Source: CAD feature listing. Evaluate the final solid. Frame: model axes, mm. A direction names the side the tool comes from. Give positions to 0.01 mm unless a question says otherwise; leave off trailing zeros. Loops run counter-clockwise (first coordinate to the right, second up) from the corner with the lowest first, then second, coordinate; pieces in that order, holes last.
from build123d import *

# Parameters (mm, degrees)
SKETCH1_R                     = 11
BOSS_BASE_FLANGE_DEPTH        = 2
BOSS_BASE_FLANGE_TAPER        = 45
SKETCH2_R                     = 9
BOSS_SPECTRA_SPOOL_DEPTH      = 13
SKETCH3_R                     = 9
BOSS_TOP_FLANGE_DEPTH         = 2
BOSS_TOP_FLANGE_DRAFT         = -45
SKETCH4_R                     = 11
BOSS_TOP_EXTENSION_DEPTH      = 8
SKETCH5_R                     = 2.6
CUT_STEPPER_SHAFT_DEPTH       = 30.444863729
CUT_SET_SCREW_HOLE_REACH      = 37.071
CUT_SET_SCREW_HOLE_END_RADIUS = 2.6
SKETCH7_R                     = 1.75
SKETCH8_R                     = 3.1
CUT_SCREW_HEAD_SLOT_DEPTH     = 2
CUT_FLATEN_REACH              = 31.445
SKETCH6_W                     = 0.753049234
SKETCH6_H                     = 8
CUT_NUT_HOLE_DEPTH            = 5
SKETCH11_W                    = 3.354551733
SKETCH11_H                    = 5.7
CUT_NUT_SLOT_DEPTH            = 5
CIRPATTERN1_COUNT             = 3
CUT_THREAD_HOLE_DEPTH         = 30.444863729
SKETCH15_W                    = 1.5
SKETCH15_H                    = 1
CUT_EXTRUDE8_DEPTH            = 28.81186797
CHAMFER1_SIZE                 = 1
CHAMFER1_SIZE2                = 0.707106781
CHAMFER3_SIZE                 = 0.3
CHAMFER3_SIZE2                = 0.519615242
SKETCH16_OUTSIDE_W            = 31.982
SKETCH16_OUTSIDE_H            = 31.982
SKETCH16_OUTSIDE_R            = 10.5
CUT_TRUNCATE_BASE_DEPTH       = 5
SKETCH8_2_R                   = 3.1
CUT_EXTRUDE9_DEPTH            = 3


with BuildPart() as part:
    # Sketch1 → Boss-Base Flange (new body)
    with BuildSketch(Plane.XY):
        Circle(SKETCH1_R)
    extrude(amount=BOSS_BASE_FLANGE_DEPTH, taper=BOSS_BASE_FLANGE_TAPER)

    # Sketch2 → Boss-Spectra Spool (add)
    with BuildSketch(Plane.XY.offset(2)):
        with Locations(Location((0, 0, 0), (0, 0, 180))):
            Circle(SKETCH2_R)
    extrude(amount=BOSS_SPECTRA_SPOOL_DEPTH)


with BuildPart() as boss_top_flange_tool:
    # Sketch3 → Boss-Top Flange (with draft: the straight prism first)
    with BuildSketch(Plane.XY.offset(15)):
        with Locations(Location((0, 0, 0), (0, 0, 180))):
            Circle(SKETCH3_R)
    extrude(amount=BOSS_TOP_FLANGE_DEPTH)
    # Boss-Top Flange: the draft: its side faces are tilted about the plane it starts from
    boss_top_flange_sides = [boss_top_flange_tool.faces().sort_by_distance(p)[0] for p in [
        (9, 0, 16),
    ]]
    draft(boss_top_flange_sides, Plane.XY.offset(15), BOSS_TOP_FLANGE_DRAFT)


with BuildPart() as part_1:
    add(part.part)

    # Boss-Top Flange: add boss_top_flange_tool
    add(boss_top_flange_tool.part)

    # Sketch4 → Boss-Top Extension (add)
    with BuildSketch(Plane.XY.offset(17)):
        Circle(SKETCH4_R)
    extrude(amount=BOSS_TOP_EXTENSION_DEPTH)

    # Sketch5 → Cut-Stepper Shaft (cut, through all)
    with BuildSketch(Plane(origin=(0, 0, 0), x_dir=(-1, 0, 0), z_dir=(0, 0, -1))):
        Circle(SKETCH5_R)
    extrude(amount=-CUT_STEPPER_SHAFT_DEPTH, mode=Mode.SUBTRACT)

    # Cut-Set Screw Hole: up to this cylinder (the profile starts outside it)
    cut_set_screw_hole_end = Plane(origin=(0, 0, 20), z_dir=(0, 0, -1)) * Cylinder(CUT_SET_SCREW_HOLE_END_RADIUS, 80.342, mode=Mode.PRIVATE)
    # Sketch7 → Cut-Set Screw Hole (cut, up to the surface)
    with BuildSketch(Plane(origin=(-11, 0, 0), x_dir=(0, 0, -1), z_dir=(1, 0, 0)), mode=Mode.PRIVATE) as cut_set_screw_hole_sk1:
        with Locations(Location((-20, 0, 0), (0, 0, 180))):
            Circle(SKETCH7_R)
    cut_set_screw_hole_tool1 = extrude(cut_set_screw_hole_sk1.sketch, amount=CUT_SET_SCREW_HOLE_REACH, mode=Mode.PRIVATE) - cut_set_screw_hole_end
    cut_set_screw_hole = cut_set_screw_hole_tool1.solids().sort_by_distance((-11, 0, 20))[0]
    add(cut_set_screw_hole, mode=Mode.SUBTRACT)

    # Sketch8 → Cut-Screw Head Slot (cut)
    with BuildSketch(Plane(origin=(-11, 0, 0), x_dir=(0, 0, -1), z_dir=(1, 0, 0))):
        with Locations(Location((-20, 0, 0), (0, 0, 194.592594316))):
            Circle(SKETCH8_R)
    cut_screw_head_slot = extrude(amount=CUT_SCREW_HEAD_SLOT_DEPTH, mode=Mode.SUBTRACT)

    # Cut-Flaten: up to this cone (the profile starts inside it)
    cut_flaten_end = Plane(origin=(0, 0, 25), z_dir=(0, 0, 1)).offset(-18.999999) * Cone(1e-06, 69.945, 69.944999, align=(Align.CENTER, Align.CENTER, Align.MIN), mode=Mode.PRIVATE)
    # Sketch6 → Cut-Flaten (cut, up to the surface)
    with BuildSketch(Plane.XY.offset(25), mode=Mode.PRIVATE) as cut_flaten_sk1:
        with Locations((-10.623475383, 0)):
            Rectangle(SKETCH6_W, SKETCH6_H)
    cut_flaten_tool1 = extrude(cut_flaten_sk1.sketch, amount=-CUT_FLATEN_REACH, mode=Mode.PRIVATE) & cut_flaten_end
    cut_flaten = cut_flaten_tool1.solids().sort_by_distance((-10.623475, 0, 25))[0]
    add(cut_flaten, mode=Mode.SUBTRACT)

    # Sketch10 → Cut-Nut Hole (cut)
    with BuildSketch(Plane.ZY):
        Polygon((23.290896534, 0), (21.645448267, 2.85), (18.354551733, 2.85), (16.709103466, 0), (18.354551733, -2.85), (21.645448267, -2.85), align=None)
    cut_nut_hole = extrude(amount=CUT_NUT_HOLE_DEPTH, mode=Mode.SUBTRACT)

    # Sketch11 → Cut-Nut Slot (cut)
    with BuildSketch(Plane.ZY):
        with Locations((23.322724134, 0)):
            Rectangle(SKETCH11_W, SKETCH11_H)
    cut_nut_slot = extrude(amount=CUT_NUT_SLOT_DEPTH, mode=Mode.SUBTRACT)

    # CirPattern1: Cut-Set Screw Hole, Cut-Screw Head Slot, Cut-Flaten, Cut-Nut Hole, Cut-Nut Slot ×3 about axis
    cirpattern1_axis = Axis((0, 0, 0), (0, 0, 1))
    add([cut_set_screw_hole.rotate(cirpattern1_axis, i * 360 / CIRPATTERN1_COUNT) for i in range(1, CIRPATTERN1_COUNT)], mode=Mode.SUBTRACT)
    add([cut_screw_head_slot.rotate(cirpattern1_axis, i * 360 / CIRPATTERN1_COUNT) for i in range(1, CIRPATTERN1_COUNT)], mode=Mode.SUBTRACT)
    add([cut_flaten.rotate(cirpattern1_axis, i * 360 / CIRPATTERN1_COUNT) for i in range(1, CIRPATTERN1_COUNT)], mode=Mode.SUBTRACT)
    add([cut_nut_hole.rotate(cirpattern1_axis, i * 360 / CIRPATTERN1_COUNT) for i in range(1, CIRPATTERN1_COUNT)], mode=Mode.SUBTRACT)
    add([cut_nut_slot.rotate(cirpattern1_axis, i * 360 / CIRPATTERN1_COUNT) for i in range(1, CIRPATTERN1_COUNT)], mode=Mode.SUBTRACT)

    # Sketch13 → Cut-Thread Hole (cut, through all)
    with BuildSketch(Plane.XY.offset(25)):
        Polygon((-4.066025404, 1), (-4.932050808, 0.5), (-4.932050808, -0.5), (-4.066025404, -1), (-3.2, -0.5), (-3.2, 0.5), align=None)
    extrude(amount=-CUT_THREAD_HOLE_DEPTH, mode=Mode.SUBTRACT)

    # Sketch15 → Cut-Extrude8 (cut, symmetric)
    with BuildSketch(Plane(origin=(-5.5, 0, 5.5), x_dir=(0.7071067811865464, 0, 0.7071067811865488), z_dir=(-0.7071067811865488, 0, 0.7071067811865464))):
        with Locations((-4.189918951, 0)):
            Rectangle(SKETCH15_W, SKETCH15_H)
    cut_extrude8 = extrude(amount=CUT_EXTRUDE8_DEPTH, both=True, mode=Mode.SUBTRACT)

    # Chamfer1
    chamfer1_edges = [part_1.edges().sort_by_distance(p)[0] for p in [
        (-4.932050808, 0, 0.067270773),
    ]]
    chamfer1_side = [part_1.faces().sort_by_distance(p)[0] for p in [
        (-6.963711629, 0, 2.098931595),
    ]]
    chamfer(chamfer1_edges, length=CHAMFER1_SIZE, length2=CHAMFER1_SIZE2, reference=chamfer1_side[0])

    # Mirror1: Cut-Extrude8 across plane
    add(cut_extrude8.mirror(Plane.XY.offset(8.5)), mode=Mode.SUBTRACT)

    # Chamfer3
    chamfer3_edges = [part_1.edges().sort_by_distance(p)[0] for p in [
        (2.6, 0, 0),
    ]]
    chamfer3_side = [part_1.faces().sort_by_distance(p)[0] for p in [
        (-10.688873016, 0, 0),
    ]]
    chamfer(chamfer3_edges, length=CHAMFER3_SIZE, length2=CHAMFER3_SIZE2, reference=chamfer3_side[0])

    # Sketch16 outside → Cut-Truncate Base (cut)
    with BuildSketch(Plane(origin=(0, 0, 0), x_dir=(-1, 0, 0), z_dir=(0, 0, -1))):
        Rectangle(SKETCH16_OUTSIDE_W, SKETCH16_OUTSIDE_H)
        Circle(SKETCH16_OUTSIDE_R, mode=Mode.SUBTRACT)
    extrude(amount=-CUT_TRUNCATE_BASE_DEPTH, mode=Mode.SUBTRACT)

    # Sketch8<2> → Cut-Extrude9 (cut)
    with BuildSketch(Plane(origin=(-11, 0, 0), x_dir=(0, 0, -1), z_dir=(1, 0, 0))):
        with Locations((-20, 0)):
            Circle(SKETCH8_2_R)
    extrude(amount=CUT_EXTRUDE9_DEPTH, mode=Mode.SUBTRACT)


solid = part_1.part
1) Reachability of faces 1 (the flat face through (-3.2, 0, 9)), 2 (the flat face through (2.535, 4.31, 22.639)), 3 (the flat face through (-7, -0.5, 16)), 4 (the cylindrical face through (-9.139, -3.066, 19.543)) from +Z, -Z, +X, -X, +Y, -Y: full face, straight path, thin tool, end or side. Return the list, or none.
Checks:
face 1: +Z, -Z
face 2: +Z
face 3: none
face 4: -X
2) Contact query for flat-ended pins moving along their axis: P1, Ø7, axis at y = 0, z = 20, coming from the -X side; P2, Ø2, axis at x = -2.5, z = 19.5, coming from the +Y side; P3, Ø2, axis at y = 4.5, z = 16.5, coming from the +X side. Output: stop coordinate, or through.
Checks:
P1: stops at x = -10.25
P2: stops at y = 10.9
P3: stops at x = 10.38
3) Pull-direction query (Y, two-part tool) for faces 5 (the flat face through (5.172, -8.846, 23.602)), 6 (the flat face through (5.075, 8.902, 23.602)), 7 (the flat face through (0.55, 3.76, 17.52)); classes: released by +Y, released by -Y, zero draft, split by the parting line, or undercut.
Checks:
face 5: released by -Y
face 6: released by +Y
face 7: undercut
4) Cut plane A-A (z = 23.5). Return loops of the section in (x, y).
Checks:
outline: (-10.25, -4) arc R11 ccw to (1.66, -10.87) - (8.59, -6.87) arc R11 ccw to (8.59, 6.87) - (1.66, 10.87) arc R11 ccw to (-10.25, 4) - close; hole (-5, -2.85) - (-1.65, -2.85) - (0.03, -5.76) - (4.97, -2.91) - (3.29, 0) - (4.97, 2.91) - (0.03, 5.76) - (-1.65, 2.85) - (-5, 2.85) - close
5) Ray query, probe 1 along Y at (x, z) = (0, 4); probe 2 along X at (y, z) = (5.5, 23.25); probe 3 along Y at (x, z) = (-9.2, 20). Return the intervals inside material, ascending.
Checks:
probe 1: y = -9 to -2.6, 2.6 to 9
probe 2: x = -9.53 to -0.12, 0.47 to 9.53
probe 3: y = -6.03 to -3.1, 3.1 to 6.03
6) Cut plane D-D (x = -6.5). State how many separate pieces and enclosed holes the cut face has, and give its area (3 significant figures).
Checks:
separate pieces: 1
enclosed holes: 2
area: 351 mm2
7) Cut plane B-B (z = 10.25). Return loops of the section in (x, y), and give its area (3 significant figures).
Checks:
outline: circle Ø18 at (0, 0); hole (-4.93, -0.5) - (-4.07, -1) - (-3.2, -0.5) - (-3.2, 0.5) - (-4.07, 1) - (-4.93, 0.5) - close; hole circle Ø5.2 at (0, 0)
area: 231 mm2
